Geometry: final body of the model. Coordinates: model frame, mm. A direction names the side the tool comes from. Coordinates: 2 decimals unless noted, no trailing zeros. Loops run counter-clockwise (first coordinate to the right, second up) from the corner with the lowest first, then second, coordinate; pieces in that order, holes last. Notation, with made-up numbers: (55.25, 77) -> (73.25, 77) arc R30 ccw to (73.25, 107) -> close; hole circle Ø2 at (68.25, 2.25). An arc over 180 degrees is marked (long way). One line per item, written item: value. Start each with the question number.
from build123d import *

# Parameters (mm, degrees)
SKETCH_1_W      = 300
SKETCH_1_H      = 200
EXTRUDE_1_DEPTH = 80
SKETCH_2_R      = 16.011496702
EXTRUDE_2_DEPTH = 20
SKETCH_3_R      = 19.343729763
EXTRUDE_3_DEPTH = 20


with BuildPart() as part:
    # 草图1 → 凸台-拉伸1 (new body)
    with BuildSketch(Plane.XY):
        Rectangle(SKETCH_1_W, SKETCH_1_H)
    extrude(amount=EXTRUDE_1_DEPTH)

    # 草图2 → 凸台-拉伸2 (add)
    with BuildSketch(Plane(origin=(0, 100, 0), x_dir=(1, 0, 0), z_dir=(0, 1, 0))):
        with Locations(Location((-100, -60, 0), (0, 0, 90))):
            Circle(SKETCH_2_R)
        with Locations(Location((100, -60, 0), (0, 0, 90))):
            Circle(SKETCH_2_R)
    extrude_2 = extrude(amount=EXTRUDE_2_DEPTH)

    # 镜向1: 凸台-拉伸2 across plane
    add(extrude_2.mirror(Plane.ZX))

    # 草图3 → 凸台-拉伸3 (add)
    with BuildSketch(Plane(origin=(0, 0, 0), x_dir=(-1, 0, 0), z_dir=(0, 0, -1))):
        with Locations((84.11011185, 0)):
            Circle(SKETCH_3_R)
    extrude(amount=EXTRUDE_3_DEPTH)


solid = part.part
1. Pin query (flat end, axial travel): pin 1 Ø8 at (x, z) = (12, 11.5) entering from +Y; pin 2 Ø4 at (x, z) = (-89.5, 25) entering from -Y; pin 3 Ø2 at (x, y) = (-119.5, 89) entering from -Z. Return the tip coordinate at first contact, or that it passes through.
2. Draft query along X for faces 1 (the face through (89.18, 109.86, 71.8)), 2 (the face through (-150, -1, 39)), 3 (the face through (100, 120, 60)). Return one class per face: released by +X, released by -X, zero draft, split by the parting line, or undercut.
3. Section B-B on x = 100. Return the cut outline in (y, z).
4. Section D-D on y = 92. Return the cut outline in (x, z).
5. Section A-A on y = 0. Return the cut outline in (x, z), plus the area to 3 significant figures.
6. Set-up query: faces 4 (the face through (-100.704, -109.86, 75.996)), 5 (the face through (-100.704, 109.86, 75.996)), 6 (the face through (-102.56, 5.81, -9.86)), 7 (the face through (-2, 1, 80)). Return all of +Z, -Z, +X, -X, +Y, -Y with unobstructed straight access to the full face (end or side cutting, diameter ignored); none if empty.
7. Line query: L1, parallel to Z at x = -122.5, y = 79; L2, parallel to Y at x = 59.5, z = 48; L3, parallel to X at y = -107.5, z = 56. Output: solid intervals per line, ascending. Write a range as [from, to].
8. Section C-C on z = 60. Return the cut outline in (x, y).
Checks:
1. pin 1: y = 100
1. pin 2: y = -100
1. pin 3: z = 0
2. face 1: undercut
2. face 2: released by -X
2. face 3: zero draft
3. outline: (-120, 43.99) -> (-100, 43.99) -> (-100, 0) -> (100, 0) -> (100, 43.99) -> (120, 43.99) -> (120, 76.01) -> (100, 76.01) -> (100, 80) -> (-100, 80) -> (-100, 76.01) -> (-120, 76.01) -> close
4. outline: (-150, 0) -> (150, 0) -> (150, 80) -> (-150, 80) -> close
5. outline: (-150, 0) -> (-103.45, 0) -> (-103.45, -20) -> (-64.77, -20) -> (-64.77, 0) -> (150, 0) -> (150, 80) -> (-150, 80) -> close
5. area: 24,800 mm²
6. face 4: -Y
6. face 5: +Y
6. face 6: -Z
6. face 7: +Z, +X, -X, +Y, -Y
7. L1: [0, 80]
7. L2: [-100, 100]
7. L3: [-115.5, -84.5], [84.5, 115.5]
8. outline: (-150, -100) -> (-116.01, -100) -> (-116.01, -120) -> (-83.99, -120) -> (-83.99, -100) -> (83.99, -100) -> (83.99, -120) -> (116.01, -120) -> (116.01, -100) -> (150, -100) -> (150, 100) -> (116.01, 100) -> (116.01, 120) -> (83.99, 120) -> (83.99, 100) -> (-83.99, 100) -> (-83.99, 120) -> (-116.01, 120) -> (-116.01, 100) -> (-150, 100) -> close
